Autodesk Inventor part; units mm, degrees
ref_plane "YZ Plane" through (0, 0, 0) normal (1, 0, 0) x (0, 1, 0)
ref_plane "XZ Plane" through (0, 0, 0) normal (0, 1, 0) x (-1, 0, 0)
ref_plane "XY Plane" through (0, 0, 0) normal (0, 0, 1) x (1, 0, 0)
sketch "Sketch1" plane through (0, 0, 0) normal (0, 0, 1) x (1, 0, 0)
  line L0 (-45, 15) -> (45, 15)
  line L1 (45, 15) -> (45, -15)
  line L2 (45, -15) -> (-45, -15)
  line L3 (-45, -15) -> (-45, 15)
  line L4 (-45, 15) -> (45, -15) construction
  line L5 (45, 15) -> (-45, -15) construction
  circle A0 centre (18, -5) radius 7.5
  circle A1 centre (-18, -5) radius 7.5
  line L6 (0, 15) -> (0, -15) construction
  line L7 (25.5, -5) -> (25.5, -15)
  line L8 (10.5, -5) -> (10.5, -15)
  line L9 (-10.5, -5) -> (-10.5, -15)
  line L10 (-25.5, -5) -> (-25.5, -15)
  line L11 (35.5, 8.8807) -> (35.5, 4.8807) construction
  line L12 (38.5, 8.8807) -> (38.5, 4.8807)
  line L13 (32.5, 4.8807) -> (32.5, 8.8807)
  arc A2 (38.5, 8.8807) -> (32.5, 8.8807) centre (35.5, 8.8807) ccw
  arc A3 (32.5, 4.8807) -> (38.5, 4.8807) centre (35.5, 4.8807) ccw
  line L14 (-35.5, 8.8807) -> (-35.5, 4.8807) construction
  line L15 (-38.5, 8.8807) -> (-38.5, 4.8807)
  line L16 (-32.5, 4.8807) -> (-32.5, 8.8807)
  arc A4 (-32.5, 8.8807) -> (-38.5, 8.8807) centre (-35.5, 8.8807) ccw
  arc A5 (-38.5, 4.8807) -> (-32.5, 4.8807) centre (-35.5, 4.8807) ccw
  point P0 (0, 0)
  point P1 (0, 0)
  point P2 (35.5, 6.8807)
  point P3 (-35.5, 6.8807)
  dimension "d0" = 90
  dimension "d1" = 30
  dimension "d2" = 15
  dimension "d3" = 36
  dimension "d6" = 10
  dimension "d7" = 6
  dimension "d8" = 4
  dimension "d9" = 71
extrude "Plate1" add sketch "Sketch1" along normal blind 2 contours L0 L1 L2 L7 A0 L8 L9 A1 L10 L3 | L10 A1 L9 L2 | L2 L8 A0 L7
fillet "Corner Round1" radius 6 4 edges at (-45, 15, 1) (-45, -15, 1) (45, 15, 1) (45, -15, 1)
equation "\"d4\" = Thickness"
equation "\"BendRadius\" = Thickness"
equation "\"BendReliefWidth\" = Thickness"
equation "\"BendReliefDepth\" = 0.5 * Thickness"
equation "\"CornerReliefSize\" = 4 * Thickness"
equation "\"MinimumRemnant\" = 2 * Thickness"
equation "\"TransitionRadius\" = BendRadius"
equation "\"JacobiRadiusSize\" = BendRadius"
equation "\"GapSize\" = Thickness"
properties part number "motor pillar 4"
The model under review builds one solid part; all positions refer to its coordinate system, in mm. A direction names the side the tool comes from. Round coordinates to 2 decimals unless told otherwise and drop trailing zeros. Order: outer loops, then holes, each group sorted by start corner. A loop starts at its lowest first (then second) coordinate and runs counter-clockwise, first axis right, second up. Notation, with made-up numbers: (-16, 75.5) -> (2, 75.5) arc R14 ccw to (2, 102.5) -> close; hole circle Ø8 at (84, 43.25). An arc over 180 degrees is marked (long way). Return JSON: item names as keys, results as strings.
1. The part is to be moulded in two halves that separate along X. For faces 3 (the face through (-43.196, 13.289, 1.014)), 4 (the face through (-1, 15, 1)), 5 (the face through (38.5, 7, 1)), 6 (the face through (35.57, 1.88, 0.99)), say which applies: +X half, -X half, draft (parallel to the pull), parting line (faces both ways), or undercut.
Answer block:
{"face 3": "-X half", "face 4": "draft", "face 5": "undercut", "face 6": "undercut"}
2. Take a section at C-C (x = -18). Write out the cut boundary in (y, z).
Answer block:
{"outline": "(-15, 0) -> (-12.5, 0) -> (-12.5, 2) -> (-15, 2) -> close; (2.5, 0) -> (15, 0) -> (15, 2) -> (2.5, 2) -> close"}
3. For faces 1 (the face through (43.289, 13.196, 1.014)), 2 (the face through (-38.5, 7, 1)), list the 3-axis set-ups (+Z, -Z, +X, -X, +Y, -Y) from which the entire face can be reached by the end or side of a thin tool; tool diameter is ignored.
Answer block:
{"face 1": "+Z, -Z, +X, +Y", "face 2": "+Z, -Z"}
4. Take a section at A-A (x = 35.5). Write out the cut boundary in (y, z), then the cut area to 3 significant figures.
Answer block:
{"outline": "(-15, 0) -> (1.88, 0) -> (1.88, 2) -> (-15, 2) -> close; (11.88, 0) -> (15, 0) -> (15, 2) -> (11.88, 2) -> close", "area": "40.0 mm²"}
5. Take a section at B-B (z = 1.5). Write out the cut boundary in (x, y).
Answer block:
{"outline": "(-45, -9) arc R6 ccw to (-39, -15) -> (39, -15) arc R6 ccw to (45, -9) -> (45, 9) arc R6 ccw to (39, 15) -> (-39, 15) arc R6 ccw to (-45, 9) -> close; hole (-38.5, 4.88) arc R3 ccw to (-32.5, 4.88) -> (-32.5, 8.88) arc R3 ccw to (-38.5, 8.88) -> close; hole circle Ø15 at (-18, -5); hole circle Ø15 at (18, -5); hole (32.5, 4.88) arc R3 ccw to (38.5, 4.88) -> (38.5, 8.88) arc R3 ccw to (32.5, 8.88) -> close"}
6. For L1, parallel to X at y = -5, z = 1.4; L2, parallel to X at y = -10.5, z = 0.4; L3, parallel to Y at x = 34, z = 1.4, list the stretches that pass through material, from the lowest coordinate up. Write a range as [from, to].
Answer block:
{"L1": "x = [-45, -25.5], [-10.5, 10.5], [25.5, 45]", "L2": "x = [-44.81, -23.1], [-12.9, 12.9], [23.1, 44.81]", "L3": "y = [-15, 2.28], [11.48, 15]"}
